The listing builds one solid part. Answer for the finished solid, in the listing's coordinates (mm). Face numbers are marked on the shaded views. A direction names the side the tool comes from. Give positions to 0.01 mm unless a question says otherwise; leave off trailing zeros. Order: outer loops, then holes, each group sorted by start corner. A loop starts at its lowest first (then second) coordinate and runs counter-clockwise, first axis right, second up. Notation, with made-up numbers: (-17.75, -7) - (17.25, -7) arc R14 cw to (17.25, 13) - close; hole circle Ø6 at (21, 50). An arc over 180 degrees is marked (long way). Use CSV: the item, a comma, the result in double quotes.
```python
from build123d import *

# Parameters (mm, degrees)
SKETCH1_W           = 12.0015
SKETCH1_H           = 9.525
BOSS_EXTRUDE3_DEPTH = 6.35
SKETCH4_W           = 38.1
SKETCH4_H           = 9.525
BOSS_EXTRUDE4_DEPTH = 22.225
SKETCH2_W           = 9.525
SKETCH2_H           = 9.525
SKETCH2_R           = 1.5875
BOSS_EXTRUDE5_DEPTH = 6.35


with BuildPart() as part:
    # Sketch1 → Boss-Extrude3 (new body)
    with BuildSketch(Plane.XY):
        with Locations((6.00075, 4.7625)):
            Rectangle(SKETCH1_W, SKETCH1_H)
    extrude(amount=-BOSS_EXTRUDE3_DEPTH)

    # Sketch4 → Boss-Extrude4 (add)
    with BuildSketch(Plane(origin=(0, 0, -6.35), x_dir=(-1, 0, 0), z_dir=(0, 0, -1))):
        with Locations((-6.00075, 4.7625)):
            Rectangle(SKETCH4_W, SKETCH4_H)
    extrude(amount=BOSS_EXTRUDE4_DEPTH)

    # Sketch2 → Boss-Extrude5 (add)
    with BuildSketch(Plane.XY):
        with Locations((-7.6835, 4.7625)):
            Rectangle(SKETCH2_W, SKETCH2_H)
        with Locations((-7.493, 4.7625)):
            Circle(SKETCH2_R, mode=Mode.SUBTRACT)
    boss_extrude5 = extrude(amount=-BOSS_EXTRUDE5_DEPTH)

    # Mirror8: Boss-Extrude5 across plane
    add(boss_extrude5.mirror(Plane(origin=(6.00075, 0, 0), x_dir=(0, 0, 1), z_dir=(1, 0, 0))))


solid = part.part
```
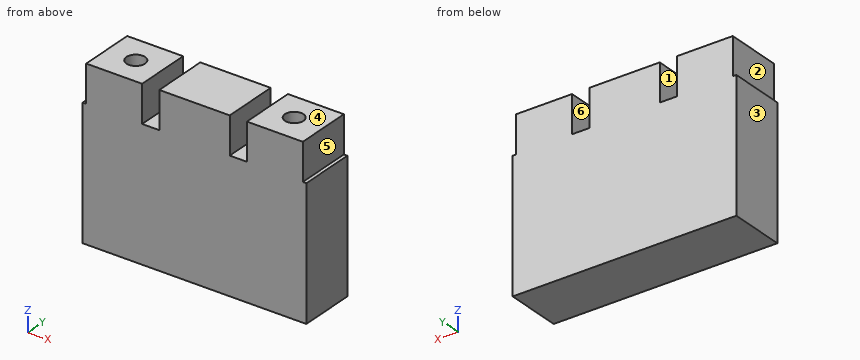
Item 1: Each of these flat-tipped pins is pushed along its axis until it touches: pin 1 (1 mm diameter, centred on x = 14.5, z = -6.5, fed in from -Y); pin 2 (0.9 mm diameter, centred on x = -2, y = 6.5, fed in from +Z); pin 3 (3 mm diameter, centred on y = 5, z = -4.5, fed in from +X). Where does it stop, or does it pass through?
Taken from the geometry:
pin 1,"y = 0"
pin 2,"z = -6.35"
pin 3,"x = 24.45"
Item 2: Find the intervals of material crossed by line 1 along X through (y, z) = (3, -5.75); line 2 along Z through (x, y) = (13, 0.5) (3 decimals), in increasing order.
Taken from the geometry:
line 1,"-12.45 to -2.92, 0 to 12, 14.92 to 24.45"
line 2,"-28.575 to -6.35"
Item 3: Which of the six approach directions +Z, -Z, +X, -X, +Y, -Y give full straight-line access (tool end or side, diameter ignored) to the marked faces 1, 2 and 3?
Taken from the geometry:
face 1,"+Z, +Y, -Y"
face 2,"+Z, -X, +Y, -Y"
face 3,"+Z, -Z, -X, +Y, -Y"
Item 4: The mould has two halves that part along X. Classify the marked faces 4, 5 and 6: +X half, -X half, draft (parallel to the pull), parting line (faces both ways), or undercut.
Taken from the geometry:
face 4,"draft"
face 5,"+X half"
face 6,"undercut"
Item 5: The part is cut by section C-C (x = -1). Give the vertices of the cut face in (y, z) (3 decimals).
Taken from the geometry:
outline,"(0, -28.575) - (9.525, -28.575) - (9.525, -6.35) - (0, -6.35) - close"
Item 6: The part is cut by section A-A (z = -2.5). Give the vertices of the cut face in (x, y) (1 decimal), and give its area (3 significant figures).
Taken from the geometry:
outline,"(-12.4, 0) - (-2.9, 0) - (-2.9, 9.5) - (-12.4, 9.5) - close; (0, 0) - (12, 0) - (12, 9.5) - (0, 9.5) - close; (14.9, 0) - (24.4, 0) - (24.4, 9.5) - (14.9, 9.5) - close; hole circle Ø3.2 at (-7.5, 4.8); hole circle Ø3.2 at (19.5, 4.8)"
area,"280 mm^2"
